Geometry check sheet. Reference: the model listing, model coordinates, mm. Give positions to 0.01 mm unless a question says otherwise; leave off trailing zeros. Loops run counter-clockwise (first coordinate to the right, second up) from the corner with the lowest first, then second, coordinate; pieces in that order, holes last.
```python
from build123d import *

# Parameters (mm, degrees)
F0_R            = 25
F0_R_2          = 3
F1_DEPTH        = 10
F3_DEPTH        = 25
F3_COPIES_COUNT = 40


# Not quite as in the source:
# - a pattern or mirror of a feature is missing from the dataset's text; its kind, count and spacing are read off the source's solid


with BuildPart() as f1:
    # F0 (on Front) → F1 (new body)
    with BuildSketch(Plane.XZ):
        Circle(F0_R)
        Circle(F0_R_2, mode=Mode.SUBTRACT)
    extrude(amount=F1_DEPTH)

    # F2 (on face) → F3 (cut)
    with BuildSketch(Plane.XZ.offset(10)):
        Polygon((2, 26), (-2, 26), (0, 20), align=None)
    f3 = extrude(amount=-F3_DEPTH, mode=Mode.SUBTRACT)

    # F3_copies: F3 ×40 about axis
    f3_copies_axis = Axis((0, 0, 0), (0, 1, 0))
    for i in range(1, F3_COPIES_COUNT):
        add(f3.rotate(f3_copies_axis, i * 360 / F3_COPIES_COUNT), mode=Mode.SUBTRACT)


solid = f1.part
```
1) Depth check by flat-ended pin: P1, Ø1, axis at y = -2.5, z = -7.5, coming from the -X side; P2, Ø4, axis at y = -5.5, z = -10, coming from the -X side; P3, Ø3, axis at y = -4.5, z = -19.5, coming from the -X side; P4, Ø5.5, axis at x = 0, z = 0, coming from the +Y side. Enter the tip coordinate at first touch or a pass-through.
2) Mould release check, pull along X, two halves, no side actions. Record for faces 1 (the flat face through (-6, -10, 0)), 2 (the flat face through (-13.91, -5.07, 17.72)): +X half, -X half, draft (parallel to the pull), parting line (faces both ways), or undercut.
3) Scan lines: line 1 along Z through (x, y) = (15, -2.25); line 2 along X through (y, z) = (-5, -16); line 3 along X through (y, z) = (-7, -19.5). Record each from-to range of solid material in increasing order.
4) Sectioned sample at A-A on x = -4. Enter the section's corners in (y, z).
Determined:
1. P1: stops at x = -21.49
1. P2: stops at x = -23.22
1. P3: stops at x = -16.47
1. P4: passes through
2. face 1: draft
2. face 2: undercut
3. line 1: z = -18.5 to -15.86, -14.57 to 14.57, 15.86 to 18.5
3. line 2: x = -19.21 to -17.86, -15.07 to 15.07, 17.86 to 19.21
3. line 3: x = -12.81 to -10.79, -9.33 to -6.53, -6.18 to 6.18, 6.53 to 9.33, 10.79 to 12.81
4. outline: (-10, -21.43) - (0, -21.43) - (0, 21.43) - (-10, 21.43) - close
